Part model, mm, in its own coordinate system. Face numbers are marked on the shaded views. A direction names the side the tool comes from. Coordinates: 2 decimals unless noted, no trailing zeros. Loops run counter-clockwise (first coordinate to the right, second up) from the corner with the lowest first, then second, coordinate; pieces in that order, holes last. Notation, with made-up numbers: (-39.5, 69.25) -> (7.5, 69.25) arc R10 ccw to (7.5, 80.25) -> close; hole circle Ø1 at (-11, 72). An arc over 180 degrees is marked (long way). Use one line per item in the form item = value. Start each with the question number.
(1) Band-saw the part on C-C on z = 15.5. Give the cut face in (x, y).
(2) 3-axis set-ups, long thin cutter, end or side, ignore diameter. For the marked faces 4 and 5: which of +Z, -Z, +X, -X, +Y, -Y reach the whole face in a straight line?
(3) Band-saw the part on B-B on x = 69.5. Give the cut face in (y, z), then the cut area to 3 significant figures.
(4) Band-saw the part on A-A on y = -20. Give the cut face in (x, z), then the cut area to 3 significant figures.
(5) Band-saw the part on D-D on x = -2. Give the cut face in (y, z), then the cut area to 3 significant figures.
(6) Mould opens along Y. For the marked faces 1, 2 and 3 say: +Y half, -Y half, draft (parallel to the pull), parting line (faces both ways), or undercut.
(7) Pin check, flat tips, straight feed: P1, Ø8.5, axis at x = -2.5, z = 2.5, coming from the -Y side; P2, Ø12, axis at x = -7, z = 18.5, coming from the -Y side; P3, Ø5, axis at x = -22.5, y = 10, coming from the +Z side. Stop position of each tip, or through.
(8) Drill centre lines: L1, parallel to Y at x = 49, z = 14; L2, parallel to Z at x = -38, y = 24; L3, parallel to X at y = 13.5, z = 11.5. Where is each one in solid material? Low to high. Write a range as [from, to].
```python
from build123d import *

# Parameters (mm, degrees)
F0_R     = 28.103341
F1_DEPTH = 38.1
F2_DEPTH = 7.62
F3_DEPTH = 30.988
F5_DEPTH = 25.4


with BuildPart() as f1:
    # F0 (on Top) → F1 (new body)
    with BuildSketch(Plane.XY):
        with BuildLine():
            ThreePointArc((88.158266, 5.448709), (68.256571, 38.830986), (29.426306, 37.198709))
            ThreePointArc((29.426306, 37.198709), (18.187712, 25.81016), (12.641991, 10.801828))
            ThreePointArc((12.641991, 10.801828), (12.262525, 5.448709), (12.641991, 0.09559))
            ThreePointArc((12.641991, 0.09559), (18.187712, -14.912741), (29.426306, -26.301291))
            ThreePointArc((29.426306, -26.301291), (68.256571, -27.933568), (88.158266, 5.448709))
        make_face()
        with Locations((50.210395, 5.448709)):
            Circle(F0_R, mode=Mode.SUBTRACT)
    extrude(amount=F1_DEPTH)

    # F0 (on Top) → F2 (join)
    with BuildSketch(Plane.XY):
        with BuildLine():
            Line((29.426306, 37.198709), (-51.389605, 37.198709))
            Line((-51.389605, 37.198709), (-51.389605, -26.301291))
            Line((-51.389605, -26.301291), (29.426306, -26.301291))
            ThreePointArc((29.426306, -26.301291), (18.187712, -14.912741), (12.641991, 0.09559))
            Line((12.641991, 0.09559), (-31.35398, 0.09559))
            Line((-31.35398, 0.09559), (-31.35398, 10.801828))
            Line((-31.35398, 10.801828), (12.641991, 10.801828))
            ThreePointArc((12.641991, 10.801828), (18.187712, 25.81016), (29.426306, 37.198709))
        make_face()
    extrude(amount=F2_DEPTH)

    # F0 (on Top) → F3 (join)
    with BuildSketch(Plane.XY):
        with BuildLine():
            ThreePointArc((12.641991, 0.09559), (12.262525, 5.448709), (12.641991, 10.801828))
            Line((12.641991, 10.801828), (-31.35398, 10.801828))
            Line((-31.35398, 10.801828), (-31.35398, 0.09559))
            Line((-31.35398, 0.09559), (12.641991, 0.09559))
        make_face()
    extrude(amount=F3_DEPTH)

    # F4 (on face) → F5 (cut)
    with BuildSketch(Plane.XZ.offset(-0.09559)):
        Polygon((-31.35398, 7.62), (12.641991, 30.988), (-31.35398, 30.988), align=None)
    extrude(amount=-F5_DEPTH, mode=Mode.SUBTRACT)


solid = f1.part
```
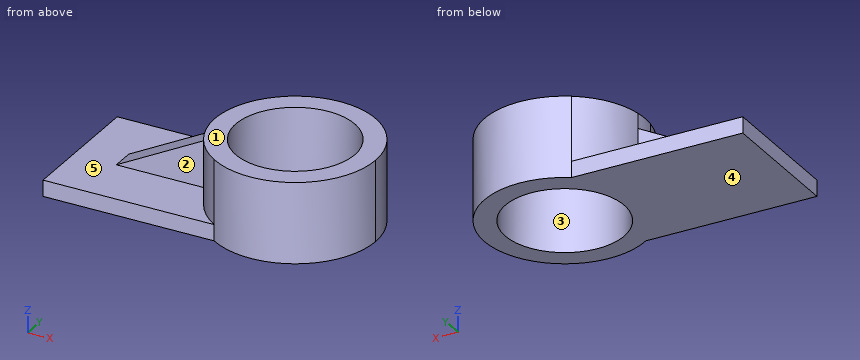
A:
q1.outline = (-16.52, 0.1) -> (12.64, 0.1) arc R37.95 ccw to (29.43, -26.3) arc R37.95 ccw (long way) to (29.43, 37.2) arc R37.95 ccw to (12.64, 10.8) -> (-16.52, 10.8) -> close; hole circle Ø56.21 at (50.21, 5.45)
q2.face_4 = -Z, +X, -X, +Y, -Y
q2.face_5 = +Z, -X
q3.outline = (-27.23, 0) -> (-14.99, 0) -> (-14.99, 38.1) -> (-27.23, 38.1) -> close; (25.89, 0) -> (38.13, 0) -> (38.13, 38.1) -> (25.89, 38.1) -> close
q3.area = 933 mm²
q4.outline = (-51.39, 0) -> (38.29, 0) -> (38.29, 38.1) -> (22.06, 38.1) -> (22.06, 7.62) -> (-51.39, 7.62) -> close; (62.13, 0) -> (78.36, 0) -> (78.36, 38.1) -> (62.13, 38.1) -> close
q4.area = 1,800 mm²
q5.outline = (-26.3, 0) -> (37.2, 0) -> (37.2, 7.62) -> (10.8, 7.62) -> (10.8, 23.21) -> (0.1, 23.21) -> (0.1, 7.62) -> (-26.3, 7.62) -> close
q5.area = 651 mm²
q6.face_1 = draft
q6.face_2 = -Y half
q6.face_3 = undercut
q7.P1 = -26.3
q7.P2 = 0.1
q7.P3 = 13.65
q8.L1 = [-32.48, -22.63], [33.53, 43.38]
q8.L2 = [0, 7.62]
q8.L3 = [13.13, 23.29], [77.14, 87.29]
